Build history of the part. All positions in model axes, mm. Face numbers are marked on the shaded views. Round coordinates to 2 decimals unless told otherwise and drop trailing zeros. Write each loop counter-clockwise with the first axis right and the second up, starting at its lowest first coordinate (ties: lowest second). Pieces come first, ordered by that corner, then holes. Notation, with made-up numbers: M 30.5,-10.75 L 39.5,-10.75 A19 ccw 39.5,18.25 Z; hole C 69.25,44.5 d1. An arc over 180 degrees is marked long. Write item = value, one per line. Start each with the question number.
Q1. Drop flat-ended pins along their axis: P1, Ø5.5, axis at x = 12.73, y = -12.73, coming from the +Z side; P2, Ø1.5, axis at x = 15.5, z = 1.5, coming from the -Y side; P3, Ø3, axis at x = -10, z = 2.5, coming from the -Y side; P4, Ø10, axis at x = 10, y = 17, coming from the -Z side. Give the stop position or say it passes through.
Q2. Band-saw the part on C-C on z = 3.95. Write the cut outline in (x, y).
Q3. Pull direction Y, two halves, no side cores. Call the marked faces 1, 2 and 3: released by +Y, released by -Y, zero draft, split by the parting line, or undercut.
Q4. Probe L1, parallel to X at y = 12, z = 4.4; L2, parallel to Y at x = -9, z = 4.6; L3, parallel to X at y = 16, z = 3.8. List the from-to ranges inside material, lowest first.
Q5. Band-saw the part on D-D on y = 12.5. State how many separate pieces and enclosed holes the cut face has, plus the area to 3 significant figures.
Q6. Band-saw the part on A-A on y = 0. Write the cut outline in (x, z).
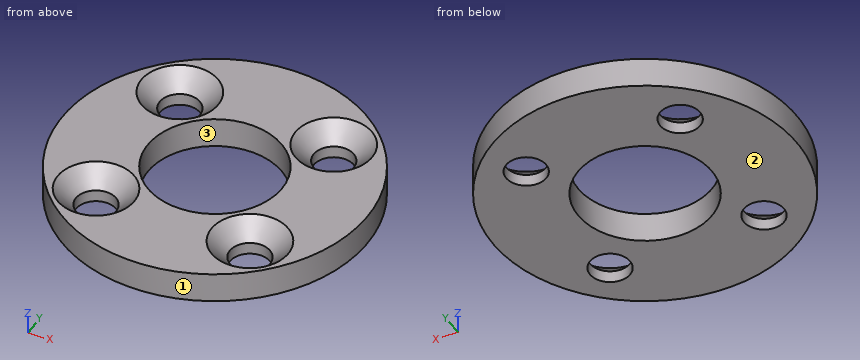
```python
from build123d import *

# Parameters (mm, degrees)
ESQUISSE1_R                                 = 25
BOSS_EXTRU_1_DEPTH                          = 5
ESQUISSE2_R                                 = 11
ENL_V_MAT_EXTRU_1_DEPTH                     = 6
FRAISAGE_POUR_VIS_T_TE_FRAIS_E_M61_AT_COUNT = 2
FRAISAGE_POUR_VIS_T_TE_FRAIS_E_M61_AT_PITCH = 36
FRAISAGE_POUR_VIS_T_TE_FRAIS_E_M61_2_COUNT  = 2
FRAISAGE_POUR_VIS_T_TE_FRAIS_E_M61_2_PITCH  = 25.455844123
FRAISAGE_POUR_VIS_T_TE_FRAIS_E_M61_3_COUNT  = 2
FRAISAGE_POUR_VIS_T_TE_FRAIS_E_M61_3_PITCH  = 25.455844123


with BuildPart() as part:
    # Esquisse1 → Boss.-Extru.1 (new body)
    with BuildSketch(Plane.XY):
        Circle(ESQUISSE1_R)
    extrude(amount=BOSS_EXTRU_1_DEPTH)

    # Esquisse2 → Enlèv. mat.-Extru.1 (cut, through all)
    with BuildSketch(Plane.XY.offset(5)):
        Circle(ESQUISSE2_R)
    extrude(amount=-ENL_V_MAT_EXTRU_1_DEPTH, mode=Mode.SUBTRACT)

    # Esquisse8 → Fraisage pour vis à tête fraisée M61 (revolve, cut)
    with BuildSketch(Plane(origin=(12.727922061, 12.727922061, 5), x_dir=(0, -1, 0), z_dir=(1, 0, 0))):
        Polygon((0, 0), (0, 5), (3.3, 5), (3.3, 3), (6.3, 0), align=None)
    fraisage_pour_vis_t_te_frais_e_m61 = revolve(axis=Axis((12.727922061, 12.727922061, 11.35), (0, 0, -1)), mode=Mode.SUBTRACT)

    # Fraisage pour vis à tête fraisée M61 at: Fraisage pour vis à tête fraisée M61 ×2
    with Locations(*[Vector(-0.707106781, -0.707106781, 0) * (i * FRAISAGE_POUR_VIS_T_TE_FRAIS_E_M61_AT_PITCH) for i in range(1, FRAISAGE_POUR_VIS_T_TE_FRAIS_E_M61_AT_COUNT)]):
        add(fraisage_pour_vis_t_te_frais_e_m61, mode=Mode.SUBTRACT)

    # Fraisage pour vis _ t_te frais_e M61 2: Fraisage pour vis à tête fraisée M61 ×2
    with Locations(*[(-i * FRAISAGE_POUR_VIS_T_TE_FRAIS_E_M61_2_PITCH, 0, 0) for i in range(1, FRAISAGE_POUR_VIS_T_TE_FRAIS_E_M61_2_COUNT)]):
        add(fraisage_pour_vis_t_te_frais_e_m61, mode=Mode.SUBTRACT)

    # Fraisage pour vis _ t_te frais_e M61 3: Fraisage pour vis à tête fraisée M61 ×2
    with Locations(*[(0, -i * FRAISAGE_POUR_VIS_T_TE_FRAIS_E_M61_3_PITCH, 0) for i in range(1, FRAISAGE_POUR_VIS_T_TE_FRAIS_E_M61_3_COUNT)]):
        add(fraisage_pour_vis_t_te_frais_e_m61, mode=Mode.SUBTRACT)


solid = part.part
```
Conclusion:
q1.P1 = through
q1.P2 = -20.19
q1.P3 = -23.51
q1.P4 = 0
q2.outline = C 0,0 d50; hole C -12.73,-12.73 d10.5; hole C -12.73,12.73 d10.5; hole C 0,0 d22; hole C 12.73,-12.73 d10.5; hole C 12.73,12.73 d10.5
q3.face_1 = split by the parting line
q3.face_2 = zero draft
q3.face_3 = undercut
q4.L1 = -21.93 to -18.38, -7.07 to 7.07, 18.38 to 21.93
q4.L2 = -23.32 to -17.3, -8.15 to -6.32, 6.32 to 8.15, 17.3 to 23.32
q4.L3 = -19.21 to -16.64, -8.82 to 8.82, 16.64 to 19.21
q5.separate_pieces = 3
q5.enclosed_holes = 0
q5.area = 133 mm^2
q6.outline = M -25,0 L -11,0 L -11,5 L -25,5 Z; M 11,0 L 25,0 L 25,5 L 11,5 Z
